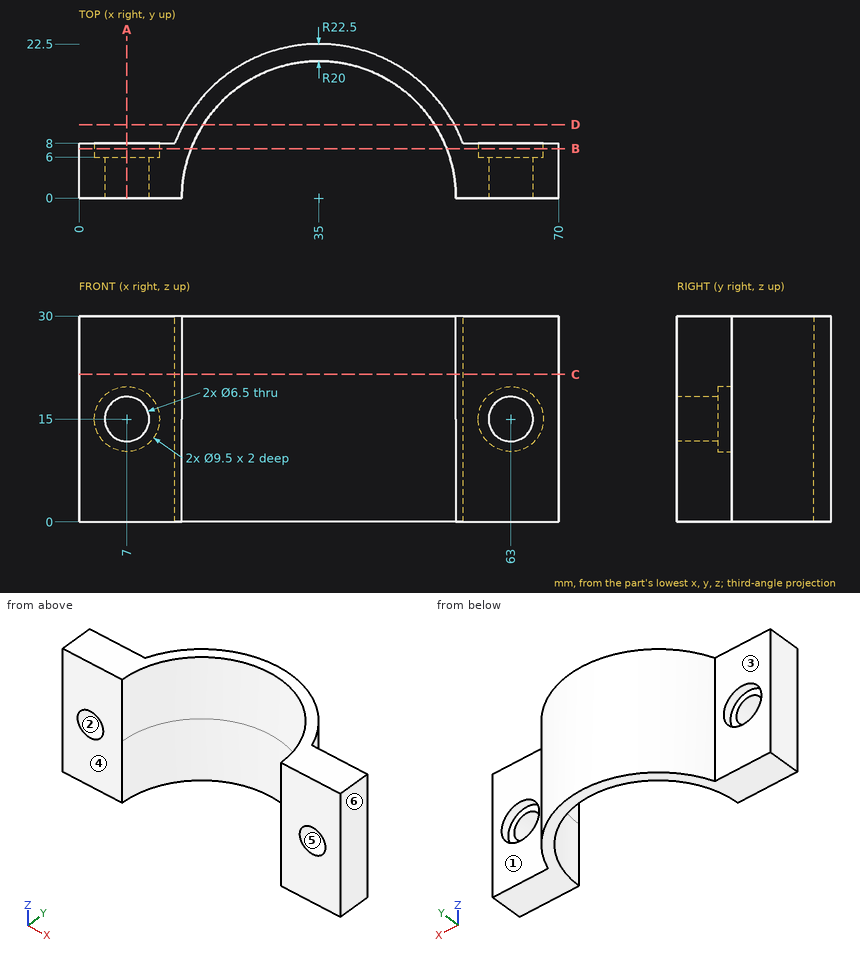
Could you check a few things on this drawing? It's one solid part, dimensions in mm from its lowest x, y, z. A direction names the side the tool comes from. Coordinates: 2 decimals unless noted, no trailing zeros. Loops run counter-clockwise (first coordinate to the right, second up) from the corner with the lowest first, then second, coordinate; pieces in that order, holes last.
1. Imagine slicing it at B-B (y = 7.25). Please give me the cut outline in (x, z), and give its area (3 significant figures).
2. We'd pull the mould along X, two halves only. Please class the marked faces 4, 5 and 6: released by +X, released by -X, zero draft, split by the parting line, or undercut.
3. I need wall thicknesses on L1, parallel to X at y = 7.5, z = 16.5; L2, parallel to Z at x = 7, y = 6.85; L3, parallel to Z at x = 7, y = 4.55. Which ranges of each line are inside material? Lowest first, please.
4. Imagine slicing it at D-D (y = 10.75). Please give me the cut outline in (x, z), and give its area (3 significant figures).
5. For the marked faces 1, 2 and 3, which set-ups out of +Z, -Z, +X, -X, +Y, -Y let a thin tool reach every point of the face, with its end or its side?
6. Imagine slicing it at C-C (z = 21.5). Please give me the cut outline in (x, y).
7. Imagine slicing it at A-A (x = 7). Please give me the cut outline in (y, z), and give its area (3 significant figures).
8. For P1, Ø6, axis at x = 47.5, z = 12, coming from the +Y side; P2, Ø8, axis at x = 15.5, z = 24.5, coming from the +Y side; P3, Ø8.5, axis at x = 63, z = 15, coming from the +Y side; P4, Ø6, axis at x = 7, z = 15, coming from the +Y side, each with a flat end and sliding along its axis, tell me the tip position at first contact or that it passes through.
Computed values:
1. outline: (0, 0) - (16.36, 0) - (16.36, 30) - (0, 30) - close; (53.64, 0) - (70, 0) - (70, 30) - (53.64, 30) - close; hole circle Ø9.5 at (7, 15); hole circle Ø9.5 at (63, 15)
1. area: 840 mm2
2. face 4: zero draft
2. face 5: undercut
2. face 6: released by +X
3. L1: x = 0 to 2.49, 11.51 to 16.46, 53.54 to 58.49, 67.51 to 70
3. L2: z = 0 to 10.25, 19.75 to 30
3. L3: z = 0 to 11.75, 18.25 to 30
4. outline: (15.23, 0) - (18.13, 0) - (18.13, 30) - (15.23, 30) - close; (51.87, 0) - (54.77, 0) - (54.77, 30) - (51.87, 30) - close
4. area: 174 mm2
5. face 1: +Z, -Z, +X, +Y
5. face 2: +Y, -Y
5. face 3: +Z, -Z, -X, +Y
6. outline: (0, 0) - (15, 0) arc R20 cw to (55, 0) - (70, 0) - (70, 8) - (56.03, 8) arc R22.5 ccw to (13.97, 8) - (0, 8) - close
7. outline: (0, 0) - (8, 0) - (8, 10.25) - (6, 10.25) - (6, 11.75) - (0, 11.75) - close; (0, 18.25) - (6, 18.25) - (6, 19.75) - (8, 19.75) - (8, 30) - (0, 30) - close
7. area: 182 mm2
8. P1: stops at y = 20.4
8. P2: stops at y = 16.31
8. P3: stops at y = 6
8. P4: passes through
